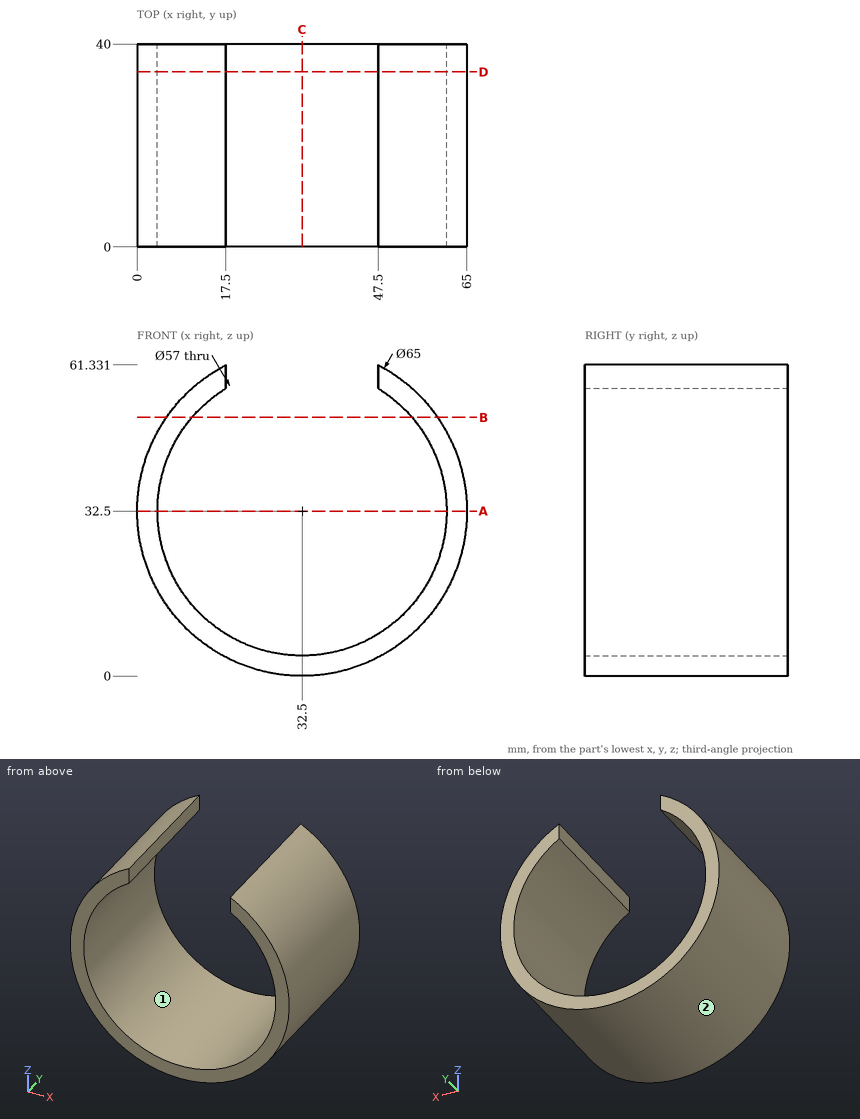
Could you check a few things on this drawing? It's one solid part, dimensions in mm from its lowest x, y, z. Coordinates: 2 decimals unless noted, no trailing zeros. Write each loop counter-clockwise with the first axis right and the second up, starting at its lowest first coordinate (ties: lowest second). Pieces come first, ordered by that corner, then holes. Notation, with made-up numbers: (-39.5, 45.25) - (6.5, 45.25) arc R14 cw to (6.5, 70.25) - close; hole circle Ø10 at (87, -36.5). An arc over 180 degrees is marked (long way). Write item = value, one per line.
1) Suppose I cut it at A-A on z = 32.5. Please give me the cut outline in (x, y), plus the area to 3 significant figures.
Result set:
outline = (0, 0) - (4, 0) - (4, 40) - (0, 40) - close; (61, 0) - (65, 0) - (65, 40) - (61, 40) - close
area = 320 mm2
2) Please list where these lines run through material, in increasing order: line 1 (X direction, y = 37, z = 33.5) (1 decimal); line 2 (Z direction, x = 32, y = 25) (1 decimal); line 3 (X direction, y = 7.5, z = 35). Write a range as [from, to].
Result set:
line_1 = [0, 4], [61, 65]
line_2 = [0, 4]
line_3 = [0.1, 4.11], [60.89, 64.9]
3) Suppose I cut it at B-B on z = 51. Please give me the cut outline in (x, y).
Result set:
outline = (5.78, 0) - (10.82, 0) - (10.82, 40) - (5.78, 40) - close; (54.18, 0) - (59.22, 0) - (59.22, 40) - (54.18, 40) - close
4) Suppose I cut it at C-C on x = 32.5. Please give me the cut outline in (y, z).
Result set:
outline = (0, 0) - (40, 0) - (40, 4) - (0, 4) - close
5) We'd pull the mould along X, two halves only. Please class the marked faces 1 and 2: +X half, -X half, draft (parallel to the pull), parting line (faces both ways), or undercut.
Result set:
face_1 = undercut
face_2 = parting line
6) Will these pins go through, and if not, where does the flat tip stop? pin 1 Ø8 at (y, z) = (31, 40.5) entering from +X; pin 2 Ø5 at (y, z) = (25, 58.5) entering from +X; pin 3 Ø5 at (y, z) = (35.5, 23) entering from -X; pin 4 Ø10 at (x, y) = (36.5, 36) entering from -Z.
Result set:
pin_1 = 64.75
pin_2 = 54.95
pin_3 = 0.76
pin_4 = 0
7) Suppose I cut it at D-D on y = 34.5. Please give me the cut outline in (x, z), plus the area to 3 significant figures.
Result set:
outline = (17.5, 56.73) - (17.5, 61.33) arc R32.5 ccw (long way) to (47.5, 61.33) - (47.5, 56.73) arc R28.5 cw (long way) to start
area = 641 mm2
